```python
from build123d import *

# Parameters (mm, degrees)
SKETCH1_R           = 12.5
BOSS_EXTRUDE1_DEPTH = 230
SKETCH2_R           = 12.5
SKETCH2_R_2         = 10
CUT_EXTRUDE1_DEPTH  = 20


with BuildPart() as part:
    # Sketch1 → Boss-Extrude1 (new body, symmetric)
    with BuildSketch(Plane(origin=(0, 0, 0), x_dir=(0, 0, -1), z_dir=(1, 0, 0))):
        Circle(SKETCH1_R)
    extrude(amount=BOSS_EXTRUDE1_DEPTH, both=True)

    # Sketch2 → Cut-Extrude1 (cut)
    with BuildSketch(Plane.ZY.offset(230)):
        Circle(SKETCH2_R)
        Circle(SKETCH2_R_2, mode=Mode.SUBTRACT)
    cut_extrude1 = extrude(amount=-CUT_EXTRUDE1_DEPTH, mode=Mode.SUBTRACT)

    # Mirror1: Cut-Extrude1 across plane
    add(cut_extrude1.mirror(Plane(origin=(0, 0, 0), x_dir=(0, 0, 1), z_dir=(1, 0, 0))), mode=Mode.SUBTRACT)


solid = part.part
```
Design review of the part built by this model. Coordinates are the model's own, in mm. A direction names the side the tool comes from. Coordinates: 2 decimals unless noted, no trailing zeros. Loops run counter-clockwise (first coordinate to the right, second up) from the corner with the lowest first, then second, coordinate; pieces in that order, holes last.
Q1. To check wall thickness, follow line 1 (Y direction, x = -88, z = -1.5); line 2 (Y direction, x = -6, z = 0); line 3 (X direction, y = -2, z = -10). State the ranges of each line that lie inside material, in increasing order.
Reported:
line 1: y = -12.41 to 12.41
line 2: y = -12.5 to 12.5
line 3: x = -210 to 210
Q2. Tool access review of faces 1 (the face through (-220.14, -9.76, -2.17)), 2 (the face through (220.14, -9.76, -2.17)), 3 (the face through (230, 0, 0)): name each direction out of +Z, -Z, +X, -X, +Y, -Y from which nothing blocks a thin tool from reaching the whole face with its end or side.
Reported:
face 1: -X
face 2: +X
face 3: +Z, -Z, +X, +Y, -Y
Q3. We need section A-A on z = 0. State the section outline as (x, y) points, and give its area (3 significant figures).
Reported:
outline: (-230, -10) - (-210, -10) - (-210, -12.5) - (210, -12.5) - (210, -10) - (230, -10) - (230, 10) - (210, 10) - (210, 12.5) - (-210, 12.5) - (-210, 10) - (-230, 10) - close
area: 11,300 mm2
Q4. We need section C-C on x = 188. State the section outline as (y, z) points.
Reported:
outline: circle Ø25 at (0, 0)
Q5. For pin 1 (1.5 mm diameter, centred on x = 38, z = 2, fed in from +Y); pin 2 (5 mm diameter, centred on x = 43.5, z = 6, fed in from +Y); pin 3 (3 mm diameter, centred on x = 175.5, y = 7, fed in from +Z) (3 decimals), all flat-tipped, find the tip position at first contact; note any pin that passes through.
Reported:
pin 1: stops at y = 12.44
pin 2: stops at y = 12
pin 3: stops at z = 11.225
